from build123d import *

# Parameters (mm, degrees)
F1_DEPTH = 29
F2_DEPTH = 18
F4_DEPTH = 27.001
F5_R     = 5


with BuildPart() as f1:
    # F0 (on Front) → F1 (new body, symmetric)
    with BuildSketch(Plane.XZ):
        with BuildLine():
            Line((0, 9), (0, 0))
            Line((0, 0), (105, 0))
            Line((105, 0), (105, 9))
            Line((105, 9), (116, 9))
            ThreePointArc((116, 9), (114.3897, 18.529129), (109.737634, 27))
            Line((109.737634, 27), (-4.737634, 27))
            ThreePointArc((-4.737634, 27), (-9.3897, 18.529129), (-11, 9))
            Line((-11, 9), (0, 9))
        make_face()
        with BuildLine():
            ThreePointArc((18, 38), (5.370669, 35.105555), (-4.737634, 27))
            Line((-4.737634, 27), (109.737634, 27))
            ThreePointArc((109.737634, 27), (99.629331, 35.105555), (87, 38))
            Line((87, 38), (18, 38))
        make_face()
    extrude(amount=F1_DEPTH, both=True)

    # F0 (on Front) → F2 (cut, symmetric)
    with BuildSketch(Plane.XZ):
        with BuildLine():
            ThreePointArc((18, 38), (5.370669, 35.105555), (-4.737634, 27))
            Line((-4.737634, 27), (109.737634, 27))
            ThreePointArc((109.737634, 27), (99.629331, 35.105555), (87, 38))
            Line((87, 38), (18, 38))
        make_face()
    extrude(amount=F2_DEPTH, both=True, mode=Mode.SUBTRACT)

    # F3 (on face) → F4 (cut, through all)
    with BuildSketch(Plane.XY.offset(27)):
        with BuildLine():
            ThreePointArc((14, 6.5), (7.5, 0), (14, -6.5))
            Line((14, -6.5), (33, -6.5))
            ThreePointArc((33, -6.5), (39.5, 0), (33, 6.5))
            Line((33, 6.5), (14, 6.5))
        make_face()
        with BuildLine():
            ThreePointArc((72, 6.5), (65.5, 0), (72, -6.5))
            Line((72, -6.5), (91, -6.5))
            ThreePointArc((91, -6.5), (97.5, 0), (91, 6.5))
            Line((91, 6.5), (72, 6.5))
        make_face()
    extrude(amount=-F4_DEPTH, mode=Mode.SUBTRACT)

    # F5
    f5_edges = [f1.edges().sort_by_distance(p)[0] for p in [
        (107.506097, -29, 29.506097),
        (107.506097, 29, 29.506097),
    ]]
    fillet(f5_edges, radius=F5_R)


solid = f1.part
The model under review builds one solid part; all positions refer to its coordinate system, in mm. A direction names the side the tool comes from. Round coordinates to 2 decimals unless told otherwise and drop trailing zeros. Loops run counter-clockwise (first coordinate to the right, second up) from the corner with the lowest first, then second, coordinate; pieces in that order, holes last. Notation, with made-up numbers: (9, -16) -> (33, -16) arc R26 ccw to (33, 6) -> close; hole circle Ø1 at (-21, -12.5). An arc over 180 degrees is marked (long way). Write item = value, one per line. Start each with the question number.
Item 1: Take a section at A-A on y = 0. Give the boundary of the cut face in (x, z), plus the area to 3 significant figures.
Item 2: Take a section at C-C on x = 46.5. Give the boundary of the cut face in (y, z), plus the area to 3 significant figures.
Item 3: For faces 1 (the flat face through (105, 0, 4)), 2 (the flat face through (24, 6.5, 14)), 3 (the flat face through (52, 0, 27)), list the 3-axis set-ups (+Z, -Z, +X, -X, +Y, -Y) from which the entire face can be reached by the end or side of a thin tool; tool diameter is ignored.
Item 4: Take a section at D-D on y = -21. Give the boundary of the cut face in (x, z), plus the area to 3 significant figures.
Item 5: Insertion check: pin 1 (12 mm diameter, centred on y = -13.5, z = 27, fed in from -X); pin 2 (10 mm diameter, centred on x = 59, y = -3.5, fed in from -Z); pin 3 (6 mm diameter, centred on y = 15.5, z = 20.5, fed in from -X); pin 4 (11 mm diameter, centred on x = 71.5, y = 3, fed in from +Z). Each pin has a flat end and moves straight along its axis. Give the tip position at first contact, or say it passes through.
Item 6: To check wall thickness, follow L1, parallel to Y at x = 84, z = 23; L2, parallel to Y at x = 41, z = 31; L3, parallel to X at y = -14, z = 5. State the ranges of each line that lie inside material, in increasing order.
Item 7: Take a section at B-B on x = 23.5. Give the boundary of the cut face in (y, z), plus the area to 3 significant figures.
Item 8: Mouldability with a two-part tool opening along X and no side actions: class faces 4 (the flat face through (52, 18, 33)), 5 (the cylindrical face through (99.794, -21.042, 35.025)), 6 (the flat face through (81, -6.5, 14)), 7 (the cylindrical face through (-9.345, -0.336, 18.657)) as released by +X, released by -X, zero draft, split by the parting line, or undercut.
Result:
q1.outline = (-11, 9) -> (0, 9) -> (0, 0) -> (7.5, 0) -> (7.5, 27) -> (-4.74, 27) arc R29 ccw to start; (39.5, 0) -> (65.5, 0) -> (65.5, 27) -> (39.5, 27) -> close; (97.5, 0) -> (105, 0) -> (105, 9) -> (116, 9) arc R29 ccw to (109.74, 27) -> (97.5, 27) -> close
q1.area = 1,430 mm²
q2.outline = (-29, 0) -> (29, 0) -> (29, 33) arc R5 ccw to (24, 38) -> (18, 38) -> (18, 27) -> (-18, 27) -> (-18, 38) -> (-24, 38) arc R5 ccw to (-29, 33) -> close
q2.area = 1,800 mm²
q3.face_1 = -Z, +X, +Y, -Y
q3.face_2 = +Z, -Z
q3.face_3 = +Z, +X, -X
q4.outline = (-11, 9) -> (0, 9) -> (0, 0) -> (105, 0) -> (105, 9) -> (116, 9) arc R29 ccw to (109.74, 27) arc R29 ccw to (87, 38) -> (18, 38) arc R29 ccw to (-4.74, 27) arc R29 ccw to start
q4.area = 4,270 mm²
q5.pin_1 = -8.4
q5.pin_2 = 0
q5.pin_3 = -9.73
q5.pin_4 = 27
q6.L1 = -29 to -6.5, 6.5 to 29
q6.L2 = -29 to -18, 18 to 29
q6.L3 = 0 to 105
q7.outline = (-29, 0) -> (-6.5, 0) -> (-6.5, 27) -> (-18, 27) -> (-18, 38) -> (-24, 38) arc R5 ccw to (-29, 33) -> close; (6.5, 0) -> (29, 0) -> (29, 33) arc R5 ccw to (24, 38) -> (18, 38) -> (18, 27) -> (6.5, 27) -> close
q7.area = 1,450 mm²
q8.face_4 = zero draft
q8.face_5 = released by +X
q8.face_6 = undercut
q8.face_7 = released by -X
